Read the model definition and answer for the solid it produces. Units are mm, in the model's axes. Face numbers are marked on the shaded views. A direction names the side the tool comes from. Coordinates: 2 decimals unless noted, no trailing zeros. Write each loop counter-clockwise with the first axis right and the second up, starting at its lowest first coordinate (ties: lowest second). Pieces come first, ordered by that corner, then holes. Notation, with made-up numbers: (57, 5) -> (79, 5) arc R16 cw to (79, 18) -> close; hole circle Ø7 at (-37.5, -26.75). An arc over 180 degrees is marked (long way). Write item = value, one per line. Start each with the question number.
1) Flat-ended cylindrical pins translate along their axes: pin 1 Ø4 at (x, z) = (19.5, 40.5) entering from -Y; pin 2 Ø1 at (x, z) = (41.5, 45) entering from +Y; pin 3 Ø3 at (x, z) = (53.5, 56) entering from +Y; pin 4 Ø6 at (y, z) = (-47, 40.5) entering from -X. Find the tip coordinate at first contact, or state that the pin passes through.
2) A tool of negligible diameter and unlimited length cuts with its end or side. For the marked faces 1, 2 and 3, from which of +Z, -Z, +X, -X, +Y, -Y can it reach the whole face along a straight path? Write none if from no direction.
3) Section A-A (y = 0) is taken. Determine the outline of the cut face in (x, z), plus the area to 3 significant figures.
4) Find the intervals of material crossed by line 1 along X through (y, z) = (41, 39.5); line 2 along Y through (x, z) = (39, 8); line 3 along Z through (x, y) = (55, -58.5), in increasing order. Write a range as from..to.
5) For a pull along Y with two mould halves and no side action, classify the marked faces 4, 5 and 6 as released by +Y, released by -Y, zero draft, split by the parting line, or undercut.
6) Section D-D (x = 6) is taken. Determine the outline of the cut face in (y, z).
7) Section B-B (x = 43.5) is taken. Determine the outline of the cut face in (y, z).
8) Section C-C (z = 29) is taken. Determine the outline of the cut face in (x, y).
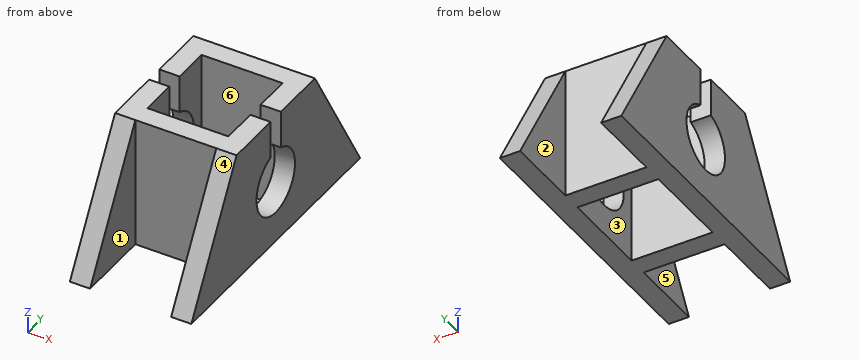
from build123d import *

# Parameters (mm, degrees)
F1_DEPTH = 60
F2_W     = 40
F2_H     = 51.5072302302
F3_DEPTH = 126
F4_W     = 40
F4_H     = 44.9444650053
F5_DEPTH = 92
F7_DEPTH = 76


with BuildPart() as f1:
    # F0 (on Right) → F1 (new body)
    with BuildSketch(Plane.YZ):
        Polygon((-70, 0), (0, 0), (70, 0), (32.4722325027, 65), (0, 65), (-32.4722325027, 65), align=None)
    extrude(amount=F1_DEPTH)

    # F2 (on face) → F3 (cut)
    with BuildSketch(Plane.XY.offset(65)):
        with Locations((30, -58.2258476178)):
            Rectangle(F2_W, F2_H)
        with Locations((30, 58.2258476178)):
            Rectangle(F2_W, F2_H)
    extrude(amount=-F3_DEPTH, mode=Mode.SUBTRACT)

    # F4 (on face) → F5 (cut)
    with BuildSketch(Plane.XY.offset(65)):
        with Locations((30, 0)):
            Rectangle(F4_W, F4_H)
    extrude(amount=-F5_DEPTH, mode=Mode.SUBTRACT)

    # F6 (on face) → F7 (cut)
    with BuildSketch(Plane.YZ.offset(60)):
        with BuildLine():
            Line((-4.2762281873, 65), (-4.2762281873, 46.3116985224))
            ThreePointArc((-4.2762281873, 46.3116985224), (0, 14.9908759852), (4.2762281873, 46.3116985224))
            Line((4.2762281873, 46.3116985224), (4.2762281873, 65))
            Line((4.2762281873, 65), (-4.2762281873, 65))
        make_face()
    extrude(amount=-F7_DEPTH, mode=Mode.SUBTRACT)


solid = f1.part
Answer key:
q1.pin_1 = -32.47
q1.pin_2 = 32.47
q1.pin_3 = 38.53
q1.pin_4 = 0
q2.face_1 = +Z, -Z, -Y
q2.face_2 = +Z, -Z, +Y
q2.face_3 = +Z, -Z
q3.outline = (0, 0) -> (10, 0) -> (10, 14.99) -> (0, 14.99) -> close; (50, 0) -> (60, 0) -> (60, 14.99) -> (50, 14.99) -> close
q3.area = 300 mm^2
q4.line_1 = 0..10, 50..60
q4.line_2 = -32.47..-22.47, 22.47..32.47
q4.line_3 = 0..19.92
q5.face_4 = released by -Y
q5.face_5 = zero draft
q5.face_6 = undercut
q6.outline = (-70, 0) -> (70, 0) -> (32.47, 65) -> (4.28, 65) -> (4.28, 46.31) arc R15.95 cw (long way) to (-4.28, 46.31) -> (-4.28, 65) -> (-32.47, 65) -> close
q7.outline = (-32.47, 0) -> (-22.47, 0) -> (-22.47, 65) -> (-32.47, 65) -> close; (22.47, 0) -> (32.47, 0) -> (32.47, 65) -> (22.47, 65) -> close
q8.outline = (0, -53.26) -> (10, -53.26) -> (10, -32.47) -> (50, -32.47) -> (50, -53.26) -> (60, -53.26) -> (60, -15.83) -> (50, -15.83) -> (50, -22.47) -> (10, -22.47) -> (10, -15.83) -> (0, -15.83) -> close; (0, 15.83) -> (10, 15.83) -> (10, 22.47) -> (50, 22.47) -> (50, 15.83) -> (60, 15.83) -> (60, 53.26) -> (50, 53.26) -> (50, 32.47) -> (10, 32.47) -> (10, 53.26) -> (0, 53.26) -> close
